Geometry check sheet. Reference: drawing and pictorial views, mm from the part's lowest x, y, z. A direction names the side the tool comes from. Round coordinates to 2 decimals unless told otherwise and drop trailing zeros. Write each loop counter-clockwise with the first axis right and the second up, starting at its lowest first coordinate (ties: lowest second). Pieces come first, ordered by that corner, then holes. Notation, with made-up numbers: (-28, 80) - (24, 80) arc R23 cw to (24, 107) - close; hole circle Ø3 at (2, 18.25). An arc over 180 degrees is marked (long way). Return JSON: item names as keys, results as strings.
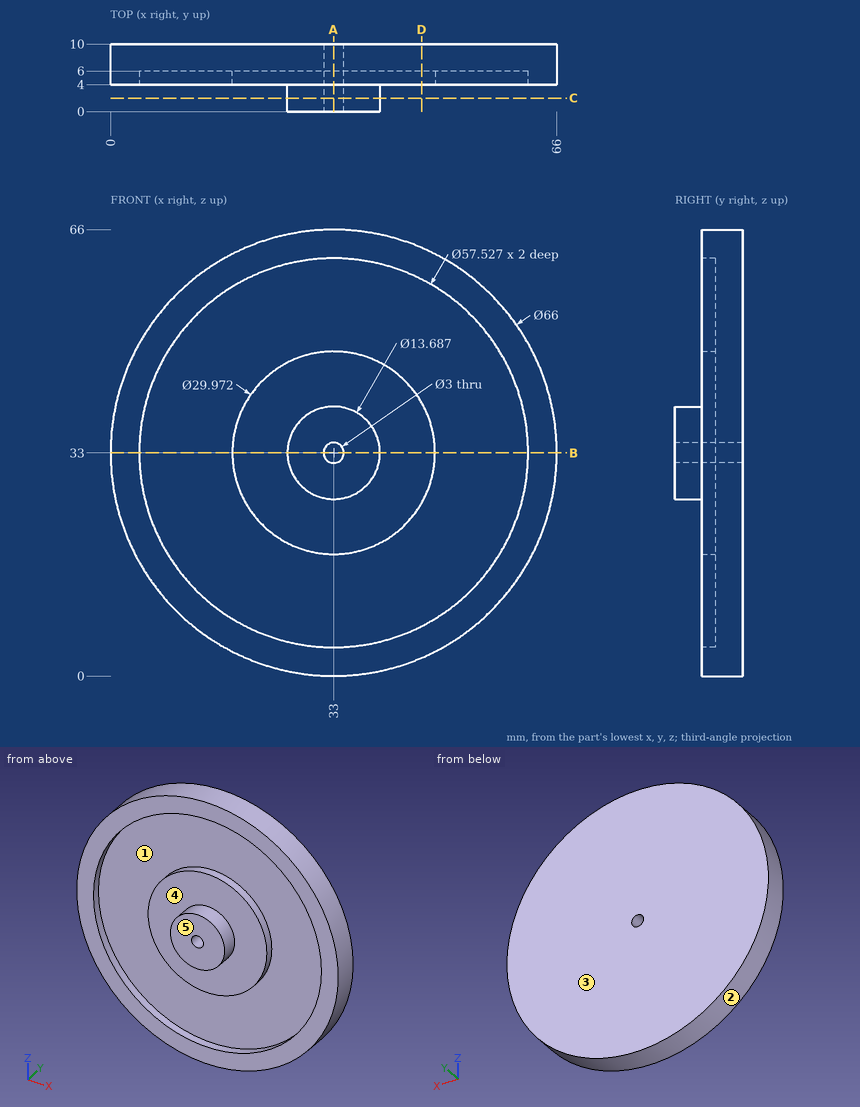
(1) Material ranges on line 1 along Z through (x, y) = (33, 4.6); line 2 along Z through (x, y) = (33, 7.5); line 3 along Y through (x, z) = (12, 32), recorded low to high. Write a range as [from, to].
Response values:
{"line 1": "z = [0, 4.24], [18.01, 31.5], [34.5, 47.99], [61.76, 66]", "line 2": "z = [0, 31.5], [34.5, 66]", "line 3": "y = [6, 10]"}
(2) Access from +Z, -Z, +X, -X, +Y, -Y to the whole of each face (thin tool, end or side, straight path). Record for the marked faces 4 and 5.
Response values:
{"face 4": "-Y", "face 5": "+Z, -Z, +X, -X, -Y"}
(3) Section check A-A, the plane x = 33. Enter the section's corners in (y, z).
Response values:
{"outline": "(0, 26.16) - (4, 26.16) - (4, 18.01) - (6, 18.01) - (6, 4.24) - (4, 4.24) - (4, 0) - (10, 0) - (10, 31.5) - (0, 31.5) - close; (0, 34.5) - (10, 34.5) - (10, 66) - (4, 66) - (4, 61.76) - (6, 61.76) - (6, 47.99) - (4, 47.99) - (4, 39.84) - (0, 39.84) - close"}
(4) Gauge pin test, flat ends, axial feed: pin 1 (1 mm diameter, centred on x = 17.5, y = 4.5, fed in from -Z); pin 2 (8 mm diameter, centred on x = 18.5, z = 13.5, fed in from -Y); pin 3 (2 mm diameter, centred on y = 2.5, z = 11, fed in from -X); pin 4 (1.5 mm diameter, centred on y = 5, z = 14.5, fed in from -X). Record the tip position at first contact, or that the pin passes through.
Response values:
{"pin 1": "stops at z = 3.61", "pin 2": "stops at y = 6", "pin 3": "passes through", "pin 4": "stops at x = 5.18"}
(5) Section check C-C, the plane y = 2. Enter the section's corners in (x, z).
Response values:
{"outline": "circle Ø13.69 at (33, 33); hole circle Ø3 at (33, 33)"}
(6) Release check for a two-part mould opening along Z. For the marked faces 1, 2 and 3 record: pulls with the +Z half, pulls with the -Z half, needs draft (parallel to the pull), parting line crosses it, or undercut.
Response values:
{"face 1": "undercut", "face 2": "parting line crosses it", "face 3": "needs draft"}
(7) Section check B-B, the plane z = 33. Enter the section's corners in (x, y).
Response values:
{"outline": "(0, 4) - (4.24, 4) - (4.24, 6) - (18.01, 6) - (18.01, 4) - (26.16, 4) - (26.16, 0) - (31.5, 0) - (31.5, 10) - (0, 10) - close; (34.5, 0) - (39.84, 0) - (39.84, 4) - (47.99, 4) - (47.99, 6) - (61.76, 6) - (61.76, 4) - (66, 4) - (66, 10) - (34.5, 10) - close"}
(8) Section check D-D, the plane x = 46. Enter the section's corners in (y, z) (1 decimal).
Response values:
{"outline": "(4, 2.7) - (10, 2.7) - (10, 63.3) - (4, 63.3) - (4, 58.7) - (6, 58.7) - (6, 40.5) - (4, 40.5) - (4, 25.5) - (6, 25.5) - (6, 7.3) - (4, 7.3) - close"}
